```python
from build123d import *

# Parameters (mm, degrees)
SHAPE_DEPTH                  = 17
SKETCH2_W                    = 14
SKETCH2_H                    = 14
THRUST_LOAD_CELL_SLOT_DEPTH  = 51.5
CHAMFER_HOLLOWING_DEPTH      = 14
SKETCH3_R                    = 2.1
THRUST_LOAD_CELL_HOLES_DEPTH = 66.749524713
SKETCH4_W                    = 14
SKETCH4_H                    = 14
TORQUE_LOAD_CELL_SLOT_DEPTH  = 27
SKETCH7_R                    = 2.1
TORQUE_LOAD_CELL_HOLES_DEPTH = 66.749524713
SKETCH8_W                    = 5
SKETCH8_H                    = 16
BOSS_EXTRUDE2_DEPTH          = 2
CUT_EXTRUDE1_DEPTH           = 15


with BuildPart() as part:
    # Sketch1 → Shape (new body)
    with BuildSketch(Plane.XY):
        Polygon((0, 0), (17, 0), (17, 27), (26, 36), (35, 36), (35, 53), (0, 53), align=None)
    extrude(amount=SHAPE_DEPTH)

    # Sketch2 → Thrust Load Cell Slot (cut)
    with BuildSketch(Plane(origin=(0, 0, 0), x_dir=(1, 0, 0), z_dir=(0, 1, 0))):
        with Locations((8.5, -8.5)):
            Rectangle(SKETCH2_W, SKETCH2_H)
    extrude(amount=THRUST_LOAD_CELL_SLOT_DEPTH, mode=Mode.SUBTRACT)

    # Sketch6 → Chamfer Hollowing (cut)
    with BuildSketch(Plane.XY.offset(1.5)):
        Polygon((25.378679656, 37.5), (15.5, 27.621320344), (15.5, 37.5), align=None)
    extrude(amount=CHAMFER_HOLLOWING_DEPTH, mode=Mode.SUBTRACT)

    # Sketch3 → Thrust Load Cell Holes (cut, through all)
    with BuildSketch(Plane(origin=(0, 0, 0), x_dir=(0, 0, -1), z_dir=(1, 0, 0))):
        with Locations((-8.5, 22)):
            Circle(SKETCH3_R)
        with Locations((-8.5, 7)):
            Circle(SKETCH3_R)
    extrude(amount=THRUST_LOAD_CELL_HOLES_DEPTH, mode=Mode.SUBTRACT)

    # Sketch4 → Torque Load Cell Slot (cut)
    with BuildSketch(Plane(origin=(35, 0, 0), x_dir=(0, 0, -1), z_dir=(1, 0, 0))):
        with Locations((-8.5, 44.5)):
            Rectangle(SKETCH4_W, SKETCH4_H)
    extrude(amount=-TORQUE_LOAD_CELL_SLOT_DEPTH, mode=Mode.SUBTRACT)

    # Sketch7 → Torque Load Cell Holes (cut, through all)
    with BuildSketch(Plane.XY):
        with Locations((6.5, 44.5)):
            Circle(SKETCH7_R)
        with Locations((21.5, 44.5)):
            Circle(SKETCH7_R)
    extrude(amount=TORQUE_LOAD_CELL_HOLES_DEPTH, mode=Mode.SUBTRACT)

    # Sketch8 → Boss-Extrude2 (add)
    with BuildSketch(Plane(origin=(0, 0, 0), x_dir=(0, 0, -1), z_dir=(1, 0, 0))):
        with Locations((-8.5, 41)):
            Rectangle(SKETCH8_W, SKETCH8_H)
    extrude(amount=-BOSS_EXTRUDE2_DEPTH)

    # Sketch9 → Cut-Extrude1 (cut)
    with BuildSketch(Plane(origin=(0, 49, 0), x_dir=(1, 0, 0), z_dir=(0, 1, 0))):
        Polygon((-2, -7.95), (-1.1, -7.95), (-1.1, -6.9), (0, -6.9), (0, -10.1), (-1.1, -10.1), (-1.1, -9.05), (-2, -9.05), align=None)
    extrude(amount=-CUT_EXTRUDE1_DEPTH, mode=Mode.SUBTRACT)


solid = part.part
```
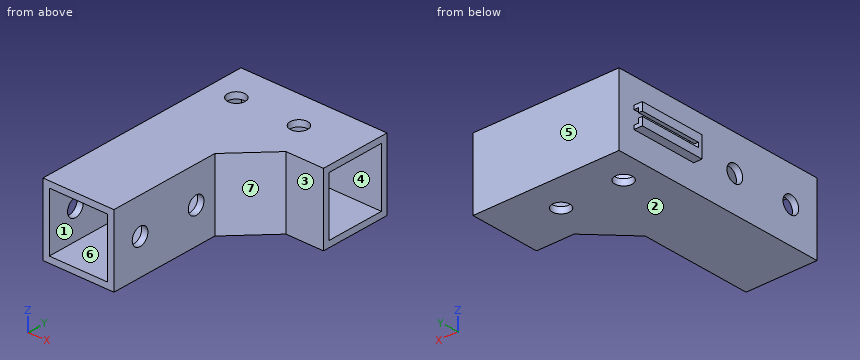
Input: part model. Units: mm. Frame: model coordinates. Face numbers are marked on the shaded views. A direction names the side the tool comes from. Give positions to 0.01 mm unless a question says otherwise; leave off trailing zeros. Order: outer loops, then holes, each group sorted by start corner. A loop starts at its lowest first (then second) coordinate and runs counter-clockwise, first axis right, second up. Notation, with made-up numbers: M 5,-10.75 L 59,-10.75 A31 ccw 59,15.25 Z; hole C -22,72 d1. An arc over 180 degrees is marked long. One line per question, with ' | ' between items. Start each with the question number.
1. First-contact query: pin 1 Ø1.2 at (x, y) = (-1, 44) entering from -Z; pin 2 Ø3 at (y, z) = (9.5, 12) entering from +X; pin 3 Ø4 at (y, z) = (16.5, 11) entering from -X; pin 4 Ø3.5 at (y, z) = (7, 8.5) entering from -X. Flat tips, straight axial feed; report the tip coordinate or a pass-through.
2. Access query for the marked faces 1, 2 and 3. Directions: +Z, -Z, +X, -X, +Y, -Y. A direction counts if a zero-diameter tool reaches every point of the face in a straight line with its end or side. Return the directions, or none.
3. Pull-direction query (Y, two-part tool) for the marked faces 4, 5, 6 and 7; classes: released by +Y, released by -Y, zero draft, split by the parting line, or undercut.
4. Section query B-B (y = 15). Return the cut outline in (x, z).
5. Material intervals for probe 1 along X at (y, z) = (44.5, 0.6); probe 2 along Z at (x, y) = (11, 50.5); probe 3 along Y at (x, z) = (33, 11.25), sorted ascending. Write a range as [from, to].
6. Section query A-A (z = 8.5). Count the separate pieces of the cut face and the enclosed holes in it, and give its area (3 significant figures).
7. Section query C-C (z = 4.75). Return the cut outline in (x, y).
8. Section query D-D (x = 6.5). Return the cut outline in (y, z), and give its area (3 significant figures).
Here are the results:
1) pin 1: z = 6 | pin 2: x = 17 | pin 3: x = 0 | pin 4: through
2) face 1: -Y | face 2: -Z, +X, -X, +Y, -Y | face 3: +Z, -Z, +X, -Y
3) face 4: undercut | face 5: released by +Y | face 6: undercut | face 7: released by -Y
4) outline: M 0,0 L 17,0 L 17,17 L 0,17 Z; hole M 1.5,1.5 L 15.5,1.5 L 15.5,15.5 L 1.5,15.5 Z
5) probe 1: [0, 4.4], [8.6, 19.4], [23.6, 35] | probe 2: [0, 1.5], [15.5, 17] | probe 3: [36, 37.5], [51.5, 53]
6) separate pieces: 6 | enclosed holes: 0 | area: 182 mm²
7) outline: M 0,0 L 1.5,0 L 1.5,51.5 L 35,51.5 L 35,53 L 0,53 Z; M 15.5,0 L 17,0 L 17,27 L 26,36 L 35,36 L 35,37.5 L 25.38,37.5 L 15.5,27.62 Z
8) outline: M 0,0 L 42.4,0 L 42.4,1.5 L 0,1.5 Z; M 0,15.5 L 42.4,15.5 L 42.4,17 L 0,17 Z; M 46.6,0 L 53,0 L 53,17 L 46.6,17 L 46.6,15.5 L 51.5,15.5 L 51.5,1.5 L 46.6,1.5 Z | area: 167 mm²
